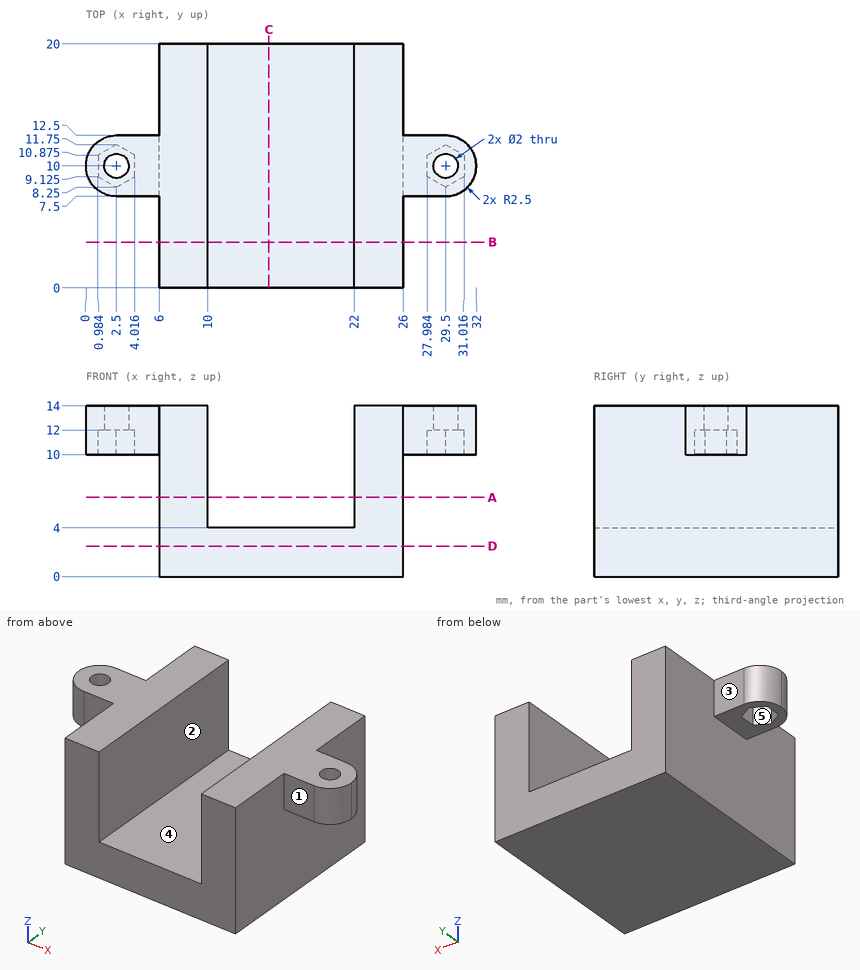
Here's the drawing with two shaded views (mm, measured from the low corner). I have some questions. A direction names the side the tool comes from. Give positions to 0.01 mm unless a question says otherwise; leave off trailing zeros. Loops run counter-clockwise (first coordinate to the right, second up) from the corner with the lowest first, then second, coordinate; pieces in that order, holes last. Notation, with made-up numbers: (77.5, -37) -> (87.5, -37) arc R24 cw to (87.5, -19) -> close; hole circle Ø9 at (44, 10). An arc over 180 degrees is marked (long way). One line per item, written item: value.
Q1. Suppose I cut it at B-B on y = 3.75. Please give me the cut outline in (x, z).
Answers follow:
outline: (6, 0) -> (26, 0) -> (26, 14) -> (22, 14) -> (22, 4) -> (10, 4) -> (10, 14) -> (6, 14) -> close
Q2. On a 3-axis mill with a long thin cutter (end or side, diameter ignored), from which of +Z, -Z, +X, -X, +Y, -Y can I reach the whole of each face in a straight line? I mean the marked faces 3, 4 and 5. Say none if no direction works.
Answers follow:
face 3: +Z, -Z, -X, +Y
face 4: +Z, +Y, -Y
face 5: -Z
Q3. Suppose I cut it at C-C on x = 15. Please give me the cut outline in (y, z).
Answers follow:
outline: (0, 0) -> (20, 0) -> (20, 4) -> (0, 4) -> close
Q4. I'm going to push flat-ended pins straight in: pin 1 Ø1.4 at (y, z) = (10.5, 11.5) entering from +X; pin 2 Ø7 at (y, z) = (9.5, 5.5) entering from -X; pin 3 Ø0.9 at (x, y) = (29, 9.5) entering from -Z; pin 4 Ø3.5 at (x, y) = (16, 7.5) entering from +Z. Where does each tip first touch, or does it pass through?
Answers follow:
pin 1: x = 32
pin 2: x = 6
pin 3: z = 12
pin 4: z = 4
Q5. Suppose I cut it at A-A on z = 6.5. Please give me the cut outline in (x, y), then the cut area to 3 significant figures.
Answers follow:
outline: (6, 0) -> (10, 0) -> (10, 20) -> (6, 20) -> close; (22, 0) -> (26, 0) -> (26, 20) -> (22, 20) -> close
area: 160 mm^2
Q6. If I drill on line 1 along X through (y, z) = (10, 13.45); line 2 along X through (y, z) = (12.25, 4.5); line 3 along Z through (x, y) = (2, 7.75), over which ranges is the centre line in solid material (lowest first)?
Answers follow:
line 1: 0 to 1.5, 3.5 to 10, 22 to 28.5, 30.5 to 32
line 2: 6 to 10, 22 to 26
line 3: 10 to 14
Q7. Suppose I cut it at D-D on z = 2.5. Please give me the cut outline in (x, y), then the cut area to 3 significant figures.
Answers follow:
outline: (6, 0) -> (26, 0) -> (26, 20) -> (6, 20) -> close
area: 400 mm^2
Q8. We'd pull the mould along X, two halves only. Please class the marked faces 1 and 2: pulls with the +X half, pulls with the -X half, needs draft (parallel to the pull), parting line crosses it, or undercut.
Answers follow:
face 1: needs draft
face 2: undercut
